from build123d import *

# Parameters (mm, degrees)
SKETCH2_R           = 1.5
BOSS_EXTRUDE1_DEPTH = 3


with BuildPart() as part:
    # Sketch2 → Boss-Extrude1 (new body)
    with BuildSketch(Plane.XY):
        with BuildLine():
            Line((-61.12281084, 10.770422233), (0.37718916, 2.976193599))
            ThreePointArc((0.37718916, 2.976193599), (1.660673927, 2.49843193), (2.598076211, 1.5))
            Line((2.598076211, 1.5), (7.098076211, -6.294228634))
            ThreePointArc((7.098076211, -6.294228634), (6.99843193, -9.454902562), (4.12281084, -10.770422233))
            Line((4.12281084, -10.770422233), (-57.37718916, -2.976193599))
            ThreePointArc((-57.37718916, -2.976193599), (-58.660673927, -2.49843193), (-59.598076211, -1.5))
            Line((-59.598076211, -1.5), (-64.098076211, 6.294228634))
            ThreePointArc((-64.098076211, 6.294228634), (-63.99843193, 9.454902562), (-61.12281084, 10.770422233))
        make_face()
        with Locations((-57, 0)):
            Circle(SKETCH2_R, mode=Mode.SUBTRACT)
        with Locations((-61.5, 7.794228634)):
            Circle(SKETCH2_R, mode=Mode.SUBTRACT)
        Circle(SKETCH2_R, mode=Mode.SUBTRACT)
        with Locations((4.5, -7.794228634)):
            Circle(SKETCH2_R, mode=Mode.SUBTRACT)
    extrude(amount=BOSS_EXTRUDE1_DEPTH)


solid = part.part
Verification items for the finished model (mm, model axes). Round coordinates to 2 decimals unless told otherwise and drop trailing zeros. Order: outer loops, then holes, each group sorted by start corner. A loop starts at its lowest first (then second) coordinate and runs counter-clockwise, first axis right, second up. Notation, with made-up numbers: (-1, 39) -> (34, 39) arc R22 ccw to (34, 66) -> close; hole circle Ø3 at (68, -32.75). An arc over 180 degrees is marked (long way). Put each result on its own line as item: value.
1) Mould release check, pull along X, two halves, no side actions. Record for faces 1 (the flat face through (-28, 0, 3)), 2 (the cylindrical face through (1.64, 2.51, 1.48)), 3 (the cylindrical face through (5.31, -6.53, 1.48)): +X half, -X half, draft (parallel to the pull), parting line (faces both ways), or undercut.
Final values:
face 1: draft
face 2: +X half
face 3: undercut
2) Material ranges on line 1 (X direction, y = 1, z = 2.7); line 2 (Y direction, x = 0, z = 1.7); line 3 (Y direction, x = -61.5, z = 0.8), recorded low to high.
Final values:
line 1: x = -61.04 to -58.12, -55.88 to -1.12, 1.12 to 2.89
line 2: y = -10.25 to -1.5, 1.5 to 3.02
line 3: y = 1.79 to 6.29, 9.29 to 10.79
3) Depth check by flat-ended pin: pin 1 (1.5 mm diameter, centred on x = -17, z = 2, fed in from -Y); pin 2 (2.5 mm diameter, centred on x = -61.5, y = 7.79, fed in from -Z). Enter the tip coordinate at first touch or a pass-through.
Final values:
pin 1: stops at y = -8.19
pin 2: passes through
4) Section check B-B (y = 0). Record the cut outline in (x, z).
Final values:
outline: (-60.46, 0) -> (-58.5, 0) -> (-58.5, 3) -> (-60.46, 3) -> close; (-55.5, 0) -> (-1.5, 0) -> (-1.5, 3) -> (-55.5, 3) -> close; (1.5, 0) -> (3.46, 0) -> (3.46, 3) -> (1.5, 3) -> close
5) Section check A-A (z = 2.2). Record the cut outline in (x, y).
Final values:
outline: (-64.1, 6.29) -> (-59.6, -1.5) arc R3 ccw to (-57.38, -2.98) -> (4.12, -10.77) arc R3 ccw to (7.1, -6.29) -> (2.6, 1.5) arc R3 ccw to (0.38, 2.98) -> (-61.12, 10.77) arc R3 ccw to start; hole circle Ø3 at (-61.5, 7.79); hole circle Ø3 at (-57, 0); hole circle Ø3 at (0, 0); hole circle Ø3 at (4.5, -7.79)
6) Section check C-C (x = -36.5). Record the cut outline in (y, z).
Final values:
outline: (-5.62, 0) -> (7.65, 0) -> (7.65, 3) -> (-5.62, 3) -> close
